Can you work these out from the model? Positions are in its coordinate system, mm. Face numbers are marked on the shaded views. Round coordinates to 2 decimals unless told otherwise and drop trailing zeros. Order: outer loops, then holes, each group sorted by start corner. A loop starts at its lowest first (then second) coordinate and runs counter-clockwise, first axis right, second up. Notation, with made-up numbers: (4, -24) - (58, -24) arc R25 ccw to (58, -10) - close; hole circle Ø1 at (87.5, 3.5). An arc over 180 degrees is marked (long way). Write item = value, one per line.
from build123d import *

# Parameters (mm, degrees)
F0_W     = 100
F0_H     = 50
F1_DEPTH = 6
F0_W_2   = 140
F0_H_2   = 90
F2_DEPTH = 3
F3_DEPTH = 3
F0_W_3   = 10
F0_H_3   = 10
F0_R     = 2.5
F4_DEPTH = 6
F5_DEPTH = 2
F6_R     = 2


with BuildPart() as f1:
    # F0 (on Top) → F1 (new body)
    with BuildSketch(Plane.XY):
        Rectangle(F0_W, F0_H)
        Polygon((-45, 10), (-45, 20), (-35, 20), (35, 20), (45, 20), (45, 10), (45, -10), (45, -20), (35, -20), (-35, -20), (-45, -20), (-45, -10), align=None, mode=Mode.SUBTRACT)
    extrude(amount=F1_DEPTH)

    # F0 (on Top) → F2 (join)
    with BuildSketch(Plane.XY):
        Rectangle(F0_W_2, F0_H_2)
        Rectangle(F0_W, F0_H, mode=Mode.SUBTRACT)
    extrude(amount=F2_DEPTH)

    # F0 (on Top) → F3 (join)
    with BuildSketch(Plane.XY):
        Rectangle(F0_W_2, F0_H_2)
        Rectangle(F0_W, F0_H, mode=Mode.SUBTRACT)
        Polygon((35, 20), (-35, 20), (-35, 10), (-45, 10), (-45, -10), (-35, -10), (-35, -20), (35, -20), (35, -10), (45, -10), (45, 10), (35, 10), align=None)
    extrude(amount=F3_DEPTH)

    # F0 (on Top) → F4 (join)
    with BuildSketch(Plane.XY):
        with Locations((-40, 15)):
            Rectangle(F0_W_3, F0_H_3)
        with Locations((-40, 15)):
            Circle(F0_R, mode=Mode.SUBTRACT)
        with Locations((40, 15)):
            Rectangle(F0_W_3, F0_H_3)
        with Locations((40, 15)):
            Circle(F0_R, mode=Mode.SUBTRACT)
        with Locations((40, -15)):
            Rectangle(F0_W_3, F0_H_3)
        with Locations((40, -15)):
            Circle(F0_R, mode=Mode.SUBTRACT)
        with Locations((-40, -15)):
            Rectangle(F0_W_3, F0_H_3)
        with Locations((-40, -15)):
            Circle(F0_R, mode=Mode.SUBTRACT)
    extrude(amount=F4_DEPTH)

    # F0 (on Top) → F5 (join)
    with BuildSketch(Plane.XY):
        with Locations((40, 15)):
            Circle(F0_R)
        with Locations((-40, 15)):
            Circle(F0_R)
        with Locations((40, -15)):
            Circle(F0_R)
        with Locations((-40, -15)):
            Circle(F0_R)
    extrude(amount=F5_DEPTH)

    # F6
    f6_edges = [f1.edges().sort_by_distance(p)[0] for p in [
        (-35, 10, 4.5),
        (35, 10, 4.5),
        (35, 20, 4.5),
        (45, 10, 4.5),
        (-35, 20, 4.5),
        (-45, 10, 4.5),
        (45, -10, 4.5),
        (35, -10, 4.5),
        (35, -20, 4.5),
        (-45, -10, 4.5),
        (-35, -10, 4.5),
        (-35, -20, 4.5),
    ]]
    fillet(f6_edges, radius=F6_R)


solid = f1.part
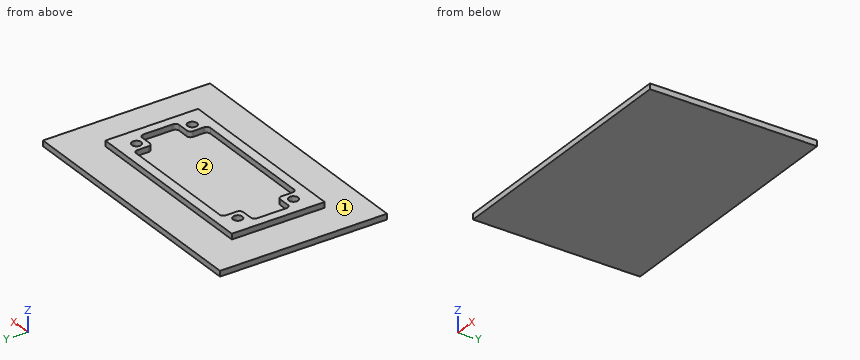
(1) If I drill on line 1 (Y direction, x = 40, z = 5.25); line 2 (Y direction, x = 43, z = 3.65); line 3 (X direction, y = -4, z = 5.35), over which ranges is the centre line in solid material (lowest first)? Write a range as from..to.
Computed:
line_1 = -25..-17.5, -12.5..-10, 10..12.5, 17.5..25
line_2 = -25..-10, 10..25
line_3 = -50..-45, 45..50
(2) If we section it at D-D (x = -24): Write out the boundary of the cut face in (y, z).
Computed:
outline = (-45, 0) - (45, 0) - (45, 3) - (25, 3) - (25, 6) - (20, 6) - (20, 3) - (-20, 3) - (-20, 6) - (-25, 6) - (-25, 3) - (-45, 3) - close
(3) Will these pins go through, and if not, where does the flat tip stop? P1, Ø3.5, axis at y = -2.5, z = 5, coming from the +X side; P2, Ø1.5, axis at x = 41, z = 4, coming from the +Y side; P3, Ø3.5, axis at y = 1, z = 5, coming from the -X side.
Computed:
P1 = 50
P2 = 25
P3 = -50
(4) Thinking about a two-plate mould opening in X: for the marked faces 1 and 2, which applies, +X half, -X half, draft (parallel to the pull), parting line (faces both ways), or undercut?
Computed:
face_1 = draft
face_2 = undercut
(5) If we section it at A-A (y = 15): Write out the boundary of the cut face in (x, z).
Computed:
outline = (-70, 0) - (70, 0) - (70, 3) - (50, 3) - (50, 6) - (42.5, 6) - (42.5, 2) - (37.5, 2) - (37.5, 6) - (35, 6) - (35, 3) - (-35, 3) - (-35, 6) - (-37.5, 6) - (-37.5, 2) - (-42.5, 2) - (-42.5, 6) - (-50, 6) - (-50, 3) - (-70, 3) - close
(6) If we section it at B-B (z = 5.05): State how many separate pieces and enclosed holes the cut face has, plus the area to 3 significant figures.
Computed:
separate_pieces = 1
enclosed_holes = 5
area = 1,720 mm^2
(7) If we section it at C-C (x = 40): Write out the boundary of the cut face in (y, z).
Computed:
outline = (-45, 0) - (45, 0) - (45, 3) - (25, 3) - (25, 6) - (17.5, 6) - (17.5, 2) - (12.5, 2) - (12.5, 6) - (10, 6) - (10, 3) - (-10, 3) - (-10, 6) - (-12.5, 6) - (-12.5, 2) - (-17.5, 2) - (-17.5, 6) - (-25, 6) - (-25, 3) - (-45, 3) - close
